from build123d import *

# Parameters (mm, degrees)
SKETCH1_W             = 140
SKETCH1_H             = 30
SKETCH1_W_2           = 35
SKETCH1_H_2           = 20
BOSS_EXTRUDE1_DEPTH   = 5
SKETCH5_W             = 41
SKETCH5_H             = 13
CUT_EXTRUDE3_DEPTH    = 3
SKETCH6_R             = 2.65
SKETCH6_R_2           = 1.35
CUT_EXTRUDE4_DEPTH    = 72.930522033
SKETCH7_R             = 2.75
CUT_EXTRUDE5_DEPTH    = 2
FILLET1_R             = 3
FILLET1_OF_MIRROR11_R = 3
FILLET2_R             = 2
CHAMFER1_SIZE         = 2.5


with BuildPart() as part:
    # Sketch1 → Boss-Extrude1 (new, symmetric)
    with BuildSketch(Plane.XY):
        Rectangle(SKETCH1_W, SKETCH1_H)
        Rectangle(SKETCH1_W_2, SKETCH1_H_2, mode=Mode.SUBTRACT)
    extrude(amount=BOSS_EXTRUDE1_DEPTH, both=True)

    # Sketch5 → Cut-Extrude3 (cut)
    with BuildSketch(Plane.XY.offset(5)):
        with Locations((-39.5, 0)):
            Rectangle(SKETCH5_W, SKETCH5_H)
    cut_extrude3 = extrude(amount=-CUT_EXTRUDE3_DEPTH, mode=Mode.SUBTRACT)

    # Sketch6 → Cut-Extrude4 (cut, through all)
    with BuildSketch(Plane.XY.offset(2)):
        with Locations((-39.5, 0)):
            Circle(SKETCH6_R)
        with Locations((-25.5, 0)):
            Circle(SKETCH6_R_2)
        with Locations(Location((-53.5, 0, 0), (0, 0, 180))):
            Circle(SKETCH6_R_2)
    cut_extrude4 = extrude(amount=-CUT_EXTRUDE4_DEPTH, mode=Mode.SUBTRACT)

    # Sketch7 → Cut-Extrude5 (cut)
    with BuildSketch(Plane(origin=(0, 0, -5), x_dir=(-1, 0, 0), z_dir=(0, 0, -1))):
        with Locations((53.5, 0)):
            Circle(SKETCH7_R)
        with Locations(Location((25.5, 0, 0), (0, 0, 180))):
            Circle(SKETCH7_R)
    cut_extrude5 = extrude(amount=-CUT_EXTRUDE5_DEPTH, mode=Mode.SUBTRACT)

    # Fillet1
    fillet1_edges = [part.edges().sort_by_distance(p)[0] for p in [
        (-42.15, 0, 2),
    ]]
    fillet(fillet1_edges, radius=FILLET1_R)

    # Mirror11: Cut-Extrude3, Cut-Extrude4, Cut-Extrude5 across plane
    add(cut_extrude3.mirror(Plane(origin=(0, 0, 0), x_dir=(0, 0, 1), z_dir=(1, 0, 0))), mode=Mode.SUBTRACT)
    add(cut_extrude4.mirror(Plane(origin=(0, 0, 0), x_dir=(0, 0, 1), z_dir=(1, 0, 0))), mode=Mode.SUBTRACT)
    add(cut_extrude5.mirror(Plane(origin=(0, 0, 0), x_dir=(0, 0, 1), z_dir=(1, 0, 0))), mode=Mode.SUBTRACT)

    # Fillet1 of Mirror11
    fillet1_of_mirror11_edges = [part.edges().sort_by_distance(p)[0] for p in [
        (42.15, 0, 2),
    ]]
    fillet(fillet1_of_mirror11_edges, radius=FILLET1_OF_MIRROR11_R)

    # Fillet2
    fillet2_edges = [part.edges().sort_by_distance(p)[0] for p in [
        (0, -15, 5),
        (0, -15, -5),
        (0, 15, -5),
        (70, -15, 0),
        (-70, -15, 0),
        (-70, 15, 0),
        (70, 15, 0),
        (0, 15, 5),
    ]]
    fillet(fillet2_edges, radius=FILLET2_R)

    # Chamfer1
    chamfer1_edges = [part.edges().sort_by_distance(p)[0] for p in [
        (17.5, -10, 0),
        (17.5, 10, 0),
        (-17.5, 10, 0),
        (-17.5, -10, 0),
    ]]
    chamfer(chamfer1_edges, length=CHAMFER1_SIZE)


solid = part.part
Check sheet for the modelled part. Datum: model origin and axes. Units: mm. A direction names the side the tool comes from. Round coordinates to 2 decimals unless told otherwise and drop trailing zeros. Order: outer loops, then holes, each group sorted by start corner. A loop starts at its lowest first (then second) coordinate and runs counter-clockwise, first axis right, second up.
(1) Draft check along X on faces 1 (the flat face through (60, 0, 4)), 2 (the flat face through (-1, 15, 0)), 3 (the cylindrical face through (50.753, 0.121, -4.014)). Enter one of: pulls with the +X half, pulls with the -X half, needs draft (parallel to the pull), parting line crosses it, or undercut.
(2) Cross-section at C-C, the plane x = -7. Enter the section's corners in (y, z), and give its area (3 significant figures).
(3) Access from +Z, -Z, +X, -X, +Y, -Y to the whole of each face (thin tool, end or side, straight path). Record for faces 4 (the flat face through (-19, 0, 4)), 5 (the flat face through (-55, 1, -3)), 6 (the flat face through (-16, -9, 0)).
(4) Go/stop test with flat-tipped pins: P1, Ø10, axis at x = 50, y = 2.5, coming from the +Z side; P2, Ø4, axis at x = -39.5, y = 0, coming from the +Z side; P3, Ø3.5, axis at x = 53.5, y = 0, coming from the +Z side; P4, Ø1.6, axis at x = -25, y = -1, coming from the -Z side. Record where each tip stops, or that it passes through.
(5) Scan lines: probe 1 along X at (y, z) = (-6.75, 1.5); probe 2 along Y at (x, z) = (53.5, -0.25); probe 3 along Y at (x, z) = (-1, 2.5). Record each from-to range of solid material in increasing order.
(6) Cross-section at B-B, the plane x = -53.5. Enter the section's corners in (y, z).
(7) Cross-section at A-A, the plane x = -39.5. Enter the section's corners in (y, z), and give its area (3 significant figures).
Check sheet entries:
1. face 1: undercut
1. face 2: needs draft
1. face 3: undercut
2. outline: (-15, -3) arc R2 ccw to (-13, -5) - (-10, -5) - (-10, 5) - (-13, 5) arc R2 ccw to (-15, 3) - close; (10, -5) - (13, -5) arc R2 ccw to (15, -3) - (15, 3) arc R2 ccw to (13, 5) - (10, 5) - close
2. area: 96.6 mm2
3. face 4: +Z
3. face 5: -Z
3. face 6: +Z, -Z
4. P1: stops at z = 5
4. P2: passes through
4. P3: stops at z = 2
4. P4: stops at z = -3
5. probe 1: x = -70 to -17.5, 17.5 to 70
5. probe 2: y = -15 to -1.35, 1.35 to 15
5. probe 3: y = -15 to -10, 10 to 15
6. outline: (-15, -3) arc R2 ccw to (-13, -5) - (-2.75, -5) - (-2.75, -3) - (-1.35, -3) - (-1.35, 2) - (-6.5, 2) - (-6.5, 5) - (-13, 5) arc R2 ccw to (-15, 3) - close; (1.35, -3) - (2.75, -3) - (2.75, -5) - (13, -5) arc R2 ccw to (15, -3) - (15, 3) arc R2 ccw to (13, 5) - (6.5, 5) - (6.5, 2) - (1.35, 2) - close
7. outline: (-15, -3) arc R2 ccw to (-13, -5) - (-2.65, -5) - (-2.65, -1) arc R3 ccw to (-5.65, 2) - (-6.5, 2) - (-6.5, 5) - (-13, 5) arc R2 ccw to (-15, 3) - close; (2.65, -5) - (13, -5) arc R2 ccw to (15, -3) - (15, 3) arc R2 ccw to (13, 5) - (6.5, 5) - (6.5, 2) - (5.65, 2) arc R3 ccw to (2.65, -1) - close
7. area: 217 mm2
